```python
from build123d import *

# Parameters (mm, degrees)
BOSS_EXTRUDE1_DEPTH = 158.75
SKETCH3_R           = 1.651
CUT_EXTRUDE1_DEPTH  = 160.825854448
SKETCH4_R           = 1.651
CUT_EXTRUDE2_DEPTH  = 160.825854448


with BuildPart() as part:
    # Sketch2 → Boss-Extrude1 (new, symmetric)
    with BuildSketch(Plane.XY):
        with BuildLine():
            Line((-9.525, -9.525), (9.525, -9.525))
            Line((9.525, -9.525), (9.525, 9.525))
            Line((9.525, 9.525), (7.9375, 9.525))
            ThreePointArc((7.9375, 9.525), (6.814967985, 9.060032015), (6.35, 7.9375))
            Line((6.35, 7.9375), (6.35, -3.175))
            ThreePointArc((6.35, -3.175), (5.42006403, -5.42006403), (3.175, -6.35))
            Line((3.175, -6.35), (-7.9375, -6.35))
            ThreePointArc((-7.9375, -6.35), (-9.060032015, -6.814967985), (-9.525, -7.9375))
            Line((-9.525, -7.9375), (-9.525, -9.525))
        make_face()
    extrude(amount=BOSS_EXTRUDE1_DEPTH, both=True)

    # Sketch3 → Cut-Extrude1 (cut, through all)
    with BuildSketch(Plane(origin=(0, -6.35, 0), x_dir=(1, 0, 0), z_dir=(0, 1, 0))):
        with Locations(Location((-2.38125, 152.4, 0), (0, 0, 180))):
            Circle(SKETCH3_R)
        with Locations(Location((-2.38125, 146.05, 0), (0, 0, 180))):
            Circle(SKETCH3_R)
        with Locations((-2.38125, -146.05)):
            Circle(SKETCH3_R)
        with Locations((-2.38125, -152.4)):
            Circle(SKETCH3_R)
    extrude(amount=-CUT_EXTRUDE1_DEPTH, mode=Mode.SUBTRACT)

    # Sketch4 → Cut-Extrude2 (cut, through all)
    with BuildSketch(Plane.ZY.offset(-6.35)):
        with Locations(Location((-152.4, 2.38125, 0), (0, 0, 270))):
            Circle(SKETCH4_R)
        with Locations(Location((-146.05, 2.38125, 0), (0, 0, 270))):
            Circle(SKETCH4_R)
        with Locations(Location((146.05, 2.38125, 0), (0, 0, 90))):
            Circle(SKETCH4_R)
        with Locations(Location((152.4, 2.38125, 0), (0, 0, 90))):
            Circle(SKETCH4_R)
    extrude(amount=-CUT_EXTRUDE2_DEPTH, mode=Mode.SUBTRACT)


solid = part.part
```
Geometry: final body of the model. Coordinates: model frame, mm. A direction names the side the tool comes from. Round coordinates to 2 decimals unless told otherwise and drop trailing zeros.
Item 1: Material intervals for L1, parallel to Y at x = 7.95, z = 152.4 (3 decimals); L2, parallel to X at y = -8, z = 146.05 (3 decimals); L3, parallel to X at y = 0, z = 56 (3 decimals), sorted ascending.
Item 2: Pin query (flat end, axial travel): P1, Ø4, axis at y = 2.38, z = -146.05, coming from the -X side; P2, Ø4.5, axis at x = -2.38, z = -146.05, coming from the +Y side; P3, Ø1, axis at y = -7, z = -61, coming from the -X side. Return the tip coordinate at first contact, or that it passes through.
Item 3: Set-up query: faces 1 (the face through (6, -6, -158.75)), 2 (the face through (6.35, 2, 2)). Return all of +Z, -Z, +X, -X, +Y, -Y with unobstructed straight access to the full face (end or side cutting, diameter ignored); none if empty.
Completed:
1. L1: y = -9.525 to 0.73, 4.032 to 9.525
1. L2: x = -9.525 to -4.032, -0.73 to 9.525
1. L3: x = 6.35 to 9.525
2. P1: stops at x = 6.35
2. P2: stops at y = -6.35
2. P3: stops at x = -9.46
3. face 1: -Z, +X, -X, +Y, -Y
3. face 2: +Z, -Z, -X, +Y
